from build123d import *

# Parameters (mm, degrees)
SKIZZE1_R                       = 3
SKIZZE1_R_2                     = 5
SKIZZE1_R_3                     = 2
AUFSATZ_LINEAR_AUSTRAGEN1_DEPTH = 10
SKIZZE2_R                       = 5
SCHNITT_LINEAR_AUSTRAGEN1_DEPTH = 4
SKIZZE3_R                       = 3
SCHNITT_LINEAR_AUSTRAGEN2_DEPTH = 5
SCHNITT_LINEAR_AUSTRAGEN3_DEPTH = 10
SKIZZE6_R                       = 1.5
SCHNITT_LINEAR_AUSTRAGEN4_DEPTH = 20
M4_GEWINDEBOHRUNG3_D            = 3.3
M4_GEWINDEBOHRUNG3_DEPTH        = 20
M4_GEWINDEBOHRUNG3_CSINK_D      = 4.05
M4_GEWINDEBOHRUNG3_CSINK_ANGLE  = 90
M4_GEWINDEBOHRUNG3_TIP          = 0.991420021


with BuildPart() as part:
    # Skizze1 → Aufsatz-Linear austragen1 (new body)
    with BuildSketch(Plane.XY):
        with BuildLine():
            Line((-28.173757618, -45.853019157), (-28.173757618, -55.229224375))
            ThreePointArc((-28.173757618, -55.229224375), (-7.173757618, -59.853019157), (13.826242382, -55.229224375))
            Line((13.826242382, -55.229224375), (13.826242382, -45.853019157))
            Line((13.826242382, -45.853019157), (13.826242382, 21.817156087))
            ThreePointArc((13.826242382, 21.817156087), (-7.173757618, 28.146980843), (-28.173757618, 21.817156087))
            Line((-28.173757618, 21.817156087), (-28.173757618, -45.853019157))
        make_face()
        with Locations((-7.173757618, -24.853019157)):
            Circle(SKIZZE1_R, mode=Mode.SUBTRACT)
        with Locations((-7.173757618, -9.853019157)):
            Circle(SKIZZE1_R_2, mode=Mode.SUBTRACT)
        with Locations((-22.673757618, -9.353019157)):
            Circle(SKIZZE1_R_3, mode=Mode.SUBTRACT)
        with Locations((-22.673757618, -40.353019157)):
            Circle(SKIZZE1_R_3, mode=Mode.SUBTRACT)
        with Locations((8.326242382, -40.353019157)):
            Circle(SKIZZE1_R_3, mode=Mode.SUBTRACT)
        with Locations((8.326242382, -9.353019157)):
            Circle(SKIZZE1_R_3, mode=Mode.SUBTRACT)
        with Locations((-7.173757618, 20.376980843)):
            Circle(SKIZZE1_R, mode=Mode.SUBTRACT)
    extrude(amount=AUFSATZ_LINEAR_AUSTRAGEN1_DEPTH)

    # Skizze2 → Schnitt-Linear austragen1 (cut)
    with BuildSketch(Plane.XY.offset(10)):
        with Locations((-7.173757618, -24.853019157)):
            Circle(SKIZZE2_R)
        with Locations((-7.173757618, 20.376980843)):
            Circle(SKIZZE2_R)
    extrude(amount=-SCHNITT_LINEAR_AUSTRAGEN1_DEPTH, mode=Mode.SUBTRACT)

    # Skizze3 → Schnitt-Linear austragen2 (cut)
    with BuildSketch(Plane(origin=(0, 0, 0), x_dir=(-1, 0, 0), z_dir=(0, 0, -1))):
        with Locations((22.694764405, -40.331983862)):
            Circle(SKIZZE3_R)
        with Locations((-8.326242382, -40.353019157)):
            Circle(SKIZZE3_R)
        with Locations((22.673757618, -9.353019157)):
            Circle(SKIZZE3_R)
        with Locations((-8.347249168, -9.374054453)):
            Circle(SKIZZE3_R)
    extrude(amount=-SCHNITT_LINEAR_AUSTRAGEN2_DEPTH, mode=Mode.SUBTRACT)

    # Skizze5 → Schnitt-Linear austragen3 (cut)
    with BuildSketch(Plane.XY.offset(10)):
        Polygon((-28.173757618, -2.226086116), (-24.173757618, 4.702117114), (-28.173757618, 7.011518191), align=None)
    extrude(amount=-SCHNITT_LINEAR_AUSTRAGEN3_DEPTH, mode=Mode.SUBTRACT)

    # Skizze6 → Schnitt-Linear austragen4 (cut)
    with BuildSketch(Plane(origin=(-20.16639465, 11.64307338, 0), x_dir=(0, 0, 1), z_dir=(-0.8660254037844384, 0.5000000000000007, 0))):
        with Locations(Location((5, -12.014725937, 0), (0, 0, 270))):
            Circle(SKIZZE6_R)
    extrude(amount=-SCHNITT_LINEAR_AUSTRAGEN4_DEPTH, mode=Mode.SUBTRACT)

    # M4 Gewindebohrung3
    with Locations(Plane(origin=(-26.173757618, 1.238015499, 5), x_dir=(-0.5, -0.866025403784, 0), z_dir=(-0.866025403784, 0.5, 0))):
        with Locations((0, 0)):
            CounterSinkHole(M4_GEWINDEBOHRUNG3_D / 2, M4_GEWINDEBOHRUNG3_CSINK_D / 2, depth=M4_GEWINDEBOHRUNG3_DEPTH, counter_sink_angle=M4_GEWINDEBOHRUNG3_CSINK_ANGLE)
            with Locations((0, 0, -(M4_GEWINDEBOHRUNG3_DEPTH + M4_GEWINDEBOHRUNG3_TIP / 2))):  # 118° drill point
                Cone(0, M4_GEWINDEBOHRUNG3_D / 2, M4_GEWINDEBOHRUNG3_TIP, mode=Mode.SUBTRACT)


solid = part.part
Work out the finished part from the listing and answer in its coordinate system (mm). A direction names the side the tool comes from. Coordinates: 2 decimals unless noted, no trailing zeros. Write each loop counter-clockwise with the first axis right and the second up, starting at its lowest first coordinate (ties: lowest second). Pieces come first, ordered by that corner, then holes. Notation, with made-up numbers: M -3.5,-30.5 L 50.5,-30.5 A29 cw 50.5,8.5 Z; hole C -33,-14.75 d7. An arc over 180 degrees is marked long. Answer as CSV lines item,"result". Start each with the question number.
Item 1: Consider L1, parallel to Y at x = -24, z = 0.5; L2, parallel to Y at x = -8.5, z = 1.5; L3, parallel to Y at x = -24, z = 7. Determine where each line is inside the solid, lowest interval first.
Item 2: A tool of negligible diameter and unlimited length cuts with its end or side. For faces 1 (the face through (-26.146, 5.841, 5.07)), 2 (the face through (-25, -10, 5)), 3 (the face through (-11.14, -27.9, 8.03)), 4 (the face through (-28.174, -28, 5)), from which of +Z, -Z, +X, -X, +Y, -Y can it reach the whole face along a straight path? Write none if from no direction.
Item 3: Section B-B on z = 1.5 is taken. Write down the section's boundary in (x, y).
Item 4: Determine the mould class of faces 5 (the face through (13.826, -17, 5)), 6 (the face through (-4.87, -14.29, 4.93)), 7 (the face through (-6.862, 28.146, 4.93)) for opening direction Y: released by +Y, released by -Y, zero draft, split by the parting line, or undercut.
Item 5: Section A-A on x = -7 is taken. Write down the section's boundary in (y, z), and give its area (3 significant figures).
Item 6: Section C-C on x = 2.5 is taken. Write down the section's boundary in (y, z).
Item 7: Flat-ended cylindrical pins translate along their axes: P1, Ø5, axis at x = 9, y = -9, coming from the -Z side; P2, Ø8, axis at x = -7.17, y = 20.38, coming from the +Z side; P3, Ø3.5, axis at x = -22.67, y = -9.35, coming from the +Z side; P4, Ø5, axis at x = 8.33, y = -40.35, coming from the -Z side. Find the tip coordinate at first contact, or state that the pin passes through.
Checks:
1,L1,"y = -56.94 to -43.03, -37.63 to -12.04, -6.66 to 24.22"
1,L2,"y = -59.84 to -27.54, -22.16 to -14.67, -5.03 to 17.69, 23.07 to 28.12"
1,L3,"y = -56.94 to -41.85, -38.86 to -10.85, -7.86 to 24.22"
2,face 1,"+Z, -Z, -X"
2,face 2,"-Z"
2,face 3,"+Z"
2,face 4,"+Z, -Z, -X, +Y, -Y"
3,outline,"M -28.17,-55.23 A50 ccw 13.83,-55.23 L 13.83,21.82 A38 ccw -28.17,21.82 L -28.17,7.01 L -24.17,4.7 L -28.17,-2.23 Z; hole C -22.69,-40.33 d6; hole C -22.67,-9.35 d6; hole C -7.17,-9.85 d10; hole C -7.17,-24.85 d6; hole C -7.17,20.38 d6; hole C 8.33,-40.35 d6; hole C 8.35,-9.37 d6"
4,face 5,"zero draft"
4,face 6,"undercut"
4,face 7,"released by +Y"
5,outline,"M -59.85,0 L -27.85,0 L -27.85,6 L -29.85,6 L -29.85,10 L -59.85,10 Z; M -21.86,0 L -14.85,0 L -14.85,10 L -19.86,10 L -19.86,6 L -21.86,6 Z; M -4.86,0 L 17.38,0 L 17.38,6 L 15.38,6 L 15.38,10 L -4.86,10 Z; M 23.37,0 L 28.15,0 L 28.15,10 L 25.37,10 L 25.37,6 L 23.37,6 Z"
5,area,"628 mm²"
6,outline,"M -58.91,0 L 26.9,0 L 26.9,10 L -58.91,10 Z"
7,P1,"stops at z = 0"
7,P2,"stops at z = 6"
7,P3,"passes through"
7,P4,"stops at z = 5"
